Geometry check sheet. Reference: drawing and pictorial views, mm from the part's lowest x, y, z. A direction names the side the tool comes from. Coordinates: 2 decimals unless noted, no trailing zeros. Loops run counter-clockwise (first coordinate to the right, second up) from the corner with the lowest first, then second, coordinate; pieces in that order, holes last. Notation, with made-up numbers: (46.5, -24.5) -> (99.5, -24.5) arc R28 cw to (99.5, 14.5) -> close; hole circle Ø3 at (-27.75, 30.5). An arc over 180 degrees is marked (long way). Answer as a JSON object with one key per item and string values.
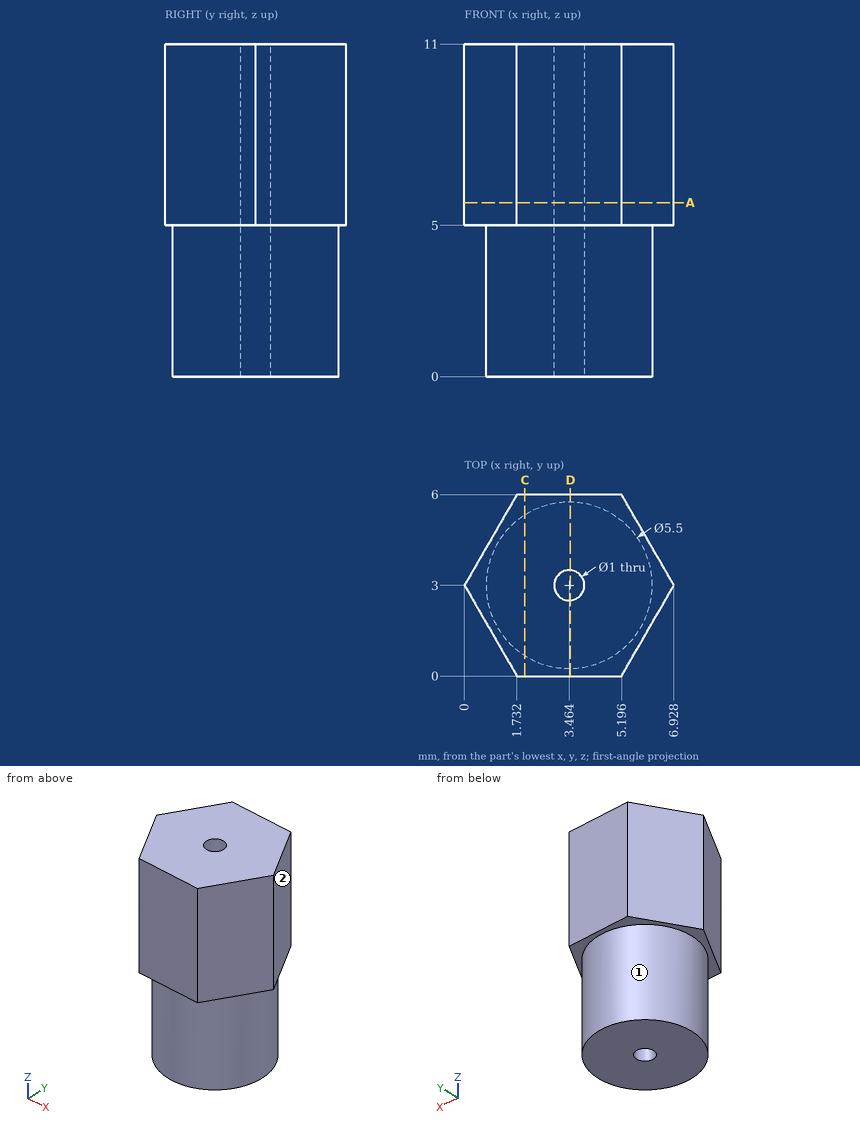
1. Tool access check on the marked faces 1 and 2. Record the directions out of +Z, -Z, +X, -X, +Y, -Y that give a thin tool (end or side, any length) a straight path to the whole face; none if there is none.
Evaluation:
{"face 1": "-Z", "face 2": "+Z, -Z, +X, +Y"}
2. Section check A-A, the plane z = 5.75. Record the boundary of the cut face in (x, y), then the cut area to 3 significant figures.
Evaluation:
{"outline": "(0, 3) -> (1.73, 0) -> (5.2, 0) -> (6.93, 3) -> (5.2, 6) -> (1.73, 6) -> close; hole circle Ø1 at (3.46, 3)", "area": "30.4 mm^2"}
3. Section check D-D, the plane x = 3.5. Record the boundary of the cut face in (y, z), then the cut area to 3 significant figures.
Evaluation:
{"outline": "(0, 5) -> (0.25, 5) -> (0.25, 0) -> (2.5, 0) -> (2.5, 11) -> (0, 11) -> close; (3.5, 0) -> (5.75, 0) -> (5.75, 5) -> (6, 5) -> (6, 11) -> (3.5, 11) -> close", "area": "52.5 mm^2"}
4. Thickness scan on probe 1 along Y at (x, z) = (3.5, 8.25); probe 2 along Z at (x, y) = (2.25, 0.5); probe 3 along X at (y, z) = (2.75, 1.25) (1 decimal). Record the ranges inside material, lowest first. Write a range as from..to.
Evaluation:
{"probe 1": "y = 0..2.5, 3.5..6", "probe 2": "z = 5..11", "probe 3": "x = 0.7..3, 3.9..6.2"}
5. Section check C-C, the plane x = 2. Record the boundary of the cut face in (y, z).
Evaluation:
{"outline": "(0, 5) -> (0.67, 5) -> (0.67, 0) -> (5.33, 0) -> (5.33, 5) -> (6, 5) -> (6, 11) -> (0, 11) -> close"}
6. Depth check by flat-ended pin: P1, Ø1, axis at x = 1, z = 5.5, coming from the -Y side; P2, Ø1.5, axis at y = 4.5, z = 1.5, coming from the -X side. Enter the tip coordinate at first touch or a pass-through.
Evaluation:
{"P1": "stops at y = 0.4", "P2": "stops at x = 0.82"}
